Work out the finished part from the listing and answer in its coordinate system (mm). A direction names the side the tool comes from. Round coordinates to 2 decimals unless told otherwise and drop trailing zeros. Write each loop counter-clockwise with the first axis right and the second up, starting at its lowest first coordinate (ties: lowest second). Pieces come first, ordered by that corner, then holes.
1. Find section A-A (y = 21). Write down the section's boundary in (x, z) (3 decimals).
2. Find section D-D (y = 39). Write down the section's boundary in (x, z) (3 decimals).
3. Find section C-C (z = 4.5). Write down the section's boundary in (x, y) (3 decimals), and give its area (3 significant figures).
4. A tool of negligible diameter and unlimited length cuts with its end or side. For faces 1 (the face through (45.8, -0.4, 38.1)), 2 (the face through (33, 25.4, 26)), 3 (the face through (-2, 7.887, 31)), 4 (the face through (-2, -7.887, 31)), from which of +Z, -Z, +X, -X, +Y, -Y can it reach the whole face along a straight path? Write none if from no direction.
5. Find section B-B (x = 71.5). Write down the section's boundary in (y, z) (1 decimal), and give its area (3 significant figures).
6. Flat-ended cylindrical pins translate along their axes: pin 1 Ø3.5 at (x, y) = (58, 1) entering from +Z; pin 2 Ø6 at (x, z) = (76.5, 44.5) entering from -Y; pin 3 Ø16.5 at (x, y) = (-12, -48) entering from +Z (3 decimals). Find the tip coordinate at first contact, or state that the pin passes through.
7. Straight lines are drawn through the part: probe 1 along Z at (x, y) = (7.5, 24) (3 decimals); probe 2 along Y at (x, z) = (-2.5, 18); probe 3 along X at (y, z) = (12.5, 14.5) (3 decimals). For each, find the intervals that lie inside material, in ascending order.
```python
from build123d import *

# Parameters (mm, degrees)
F1_DEPTH    = 63.5
F0_W        = 25.4
F0_H        = 19.05
F0_H_2      = 4.7498
F0_H_3      = 4.7752
F2_DEPTH    = 25.4
F3_DEPTH    = 7.8867
F5_T1_DEPTH = 124.7474881183
F5_T3_DEPTH = 88.9
F5_T6_ANGLE = 180


# Not quite as in the source:
# - a fillet or chamfer that OpenCascade refuses, or shapes differently, is made with other operations: its cross-section is extruded or revolved along the edge and cut away or added


with BuildPart() as f1:
    # F0 (on Front) → F1 (new body, symmetric)
    with BuildSketch(Plane.XZ):
        Polygon((22.225, 9.525), (-41.275, 9.525), (-41.275, -9.525), (41.275, -9.525), (41.275, 9.525), align=None)
    extrude(amount=F1_DEPTH, both=True)

    # F0 (on Front) → F2 (join, symmetric)
    with BuildSketch(Plane.XZ):
        with BuildLine():
            Line((22.225, 27.0002), (22.225, 9.525))
            Line((22.225, 9.525), (41.275, 9.525))
            Line((41.275, 9.525), (41.275, 27.0002))
            ThreePointArc((41.275, 27.0002), (45.9246798487, 38.2255201513), (57.15, 42.8752))
            Line((57.15, 42.8752), (60.325, 42.8752))
            Line((60.325, 42.8752), (60.325, 61.9252))
            Line((60.325, 61.9252), (57.15, 61.9252))
            ThreePointArc((57.15, 61.9252), (32.4542956671, 51.6959043329), (22.225, 27.0002))
        make_face()
        with Locations((73.025, 52.4002)):
            Rectangle(F0_W, F0_H)
        with Locations((73.025, 64.3001)):
            Rectangle(F0_W, F0_H_2)
        with Locations((73.025, 40.4876)):
            Rectangle(F0_W, F0_H_3)
    extrude(amount=F2_DEPTH, both=True)

    # F0 (on Front) → F3 (join, symmetric)
    with BuildSketch(Plane.XZ):
        with BuildLine():
            add(Edge.make_bspline(
                [(-41.275, 9.525), (-41.0557202995, 48.5295318067), (2.8826263733, 65.0303959846), (57.15, 61.9252)],
                knots=[0, 0, 0, 0, 111.5045361635, 111.5045361635, 111.5045361635, 111.5045361635], degree=3))
            Line((-41.275, 9.525), (22.225, 9.525))
            Line((22.225, 9.525), (22.225, 27.0002))
            ThreePointArc((22.225, 27.0002), (32.4542956671, 51.6959043329), (57.15, 61.9252))
        make_face()
    extrude(amount=F3_DEPTH, both=True)

    # F0 (on Front) → F4 (revolve)
    with BuildSketch(Plane.XZ):
        Polygon((85.725, 66.675), (85.725, 61.9252), (85.725, 42.8752), (85.725, 38.1), (111.125, 38.1), (111.125, 66.675), align=None)
    revolve(axis=Axis((85.725, 0, 52.3875), (0, 0, 1)))

    # F5: fillet of radius 25.4 on 4 edges, made by hand

    # F5_s2 → F5_t1 (cut)
    with BuildSketch(Plane.XZ.offset(-62.3737440591)):
        with BuildLine():
            ThreePointArc((60.325, 61.9252), (67.3477441191, 65.4584145645), (75.1144976237, 66.675))
            Line((75.1144976237, 66.675), (60.325, 66.675))
            Line((60.325, 66.675), (60.325, 61.9252))
        make_face()
    extrude(amount=F5_T1_DEPTH, mode=Mode.SUBTRACT)

    # F5_s4 → F5_t3 (cut)
    with BuildSketch(Plane.YZ.offset(-3.175)):
        with BuildLine():
            ThreePointArc((-25.4, 41.275), (-17.9605122421, 59.2355122421), (0, 66.675))
            Line((0, 66.675), (-25.4, 66.675))
            Line((-25.4, 66.675), (-25.4, 41.275))
        make_face()
        with BuildLine():
            ThreePointArc((0, 66.675), (17.9605122421, 59.2355122421), (25.4, 41.275))
            Line((25.4, 41.275), (25.4, 66.675))
            Line((25.4, 66.675), (0, 66.675))
        make_face()
    extrude(amount=F5_T3_DEPTH, mode=Mode.SUBTRACT)

    # F5_s5 → F5_t6 (revolve, cut)
    with BuildSketch(Plane.YZ.offset(85.725)):
        with BuildLine():
            ThreePointArc((0, 66.675), (17.9605122421, 59.2355122421), (25.4, 41.275))
            Line((25.4, 41.275), (25.4, 66.675))
            Line((25.4, 66.675), (0, 66.675))
        make_face()
    revolve(axis=Axis((85.725, 0, 66.675), (0, 0, -1)), revolution_arc=F5_T6_ANGLE, mode=Mode.SUBTRACT)


solid = f1.part
```
Worked answers:
1. outline: (-41.275, -9.525) - (41.275, -9.525) - (41.275, 27) arc R15.875 cw to (57.15, 42.875) - (60.325, 42.875) - (60.325, 38.1) - (100.013, 38.1) - (100.013, 41.275) arc R14.288 ccw to (85.725, 55.563) - (37.053, 55.563) arc R34.925 ccw to (22.225, 27) - (22.225, 9.525) - (-41.275, 9.525) - close
2. outline: (-41.275, -9.525) - (41.275, -9.525) - (41.275, 9.525) - (-41.275, 9.525) - close
3. outline: (-41.275, -63.5) - (41.275, -63.5) - (41.275, 63.5) - (-41.275, 63.5) - close
3. area: 10,500 mm2
4. face 1: -Z, +Y, -Y
4. face 2: +Z, +X, -X, +Y
4. face 3: +Z, -X, +Y
4. face 4: +Z, -X, -Y
5. outline: (-25.4, 38.1) - (25.4, 38.1) - (25.4, 41.3) arc R25.4 ccw to (3.6, 66.4) - (-3.6, 66.4) arc R25.4 ccw to (-25.4, 41.3) - close
5. area: 1,170 mm2
6. pin 1: stops at z = 61.97
6. pin 2: stops at y = -25.4
6. pin 3: stops at z = 9.525
7. probe 1: z = -9.525 to 9.525
7. probe 2: y = -7.89 to 7.89
7. probe 3: x = 22.225 to 41.275
